Build history of the part. All positions in model axes, mm. Face numbers are marked on the shaded views. A direction names the side the tool comes from. Round coordinates to 2 decimals unless told otherwise and drop trailing zeros. Write each loop counter-clockwise with the first axis right and the second up, starting at its lowest first coordinate (ties: lowest second). Pieces come first, ordered by that corner, then holes.
Item 1: Drop flat-ended pins along their axis: pin 1 Ø1.5 at (y, z) = (11.5, 3) entering from -X; pin 2 Ø12 at (x, y) = (3, 0) entering from -Z; pin 3 Ø1.5 at (y, z) = (10, 2.5) entering from +X; pin 4 Ø1.5 at (x, y) = (11, -4) entering from +Z. Give the stop position or say it passes through.
Item 2: Wall check: probe 1 along Y at (x, z) = (-10, 2.1); probe 2 along Y at (x, z) = (-8, 0.4); probe 3 along X at (y, z) = (-10, 2.45). Give the ranges that are in metal, low to high.
Item 3: Band-saw the part on C-C, the plane x = 22.5. Write the cut outline in (y, z).
Item 4: Band-saw the part on A-A, the plane y = -9.5. Write the cut outline in (x, z).
Item 5: 3-axis set-ups, long thin cutter, end or side, ignore diameter. For the marked faces 4 and 5: which of +Z, -Z, +X, -X, +Y, -Y reach the whole face in a straight line?
Item 6: Band-saw the part on B-B, the plane x = 6. Write the cut outline in (y, z), then the cut area to 3 significant figures.
Item 7: Mould opens along X. For the marked faces 1, 2 and 3 say: +X half, -X half, draft (parallel to the pull), parting line (faces both ways), or undercut.
Item 8: Band-saw the part on D-D, the plane z = 2.5. Count the separate pieces of the cut face and the enclosed holes in it, then the cut area to 3 significant figures.
```python
from build123d import *

# Parameters (mm, degrees)
SKETCH1_W                 = 42
SKETCH1_H                 = 43
BOSS_EXTRUDE1_DEPTH       = 5
SKETCH2_W                 = 31.6
SKETCH2_H                 = 12.6
CUT_EXTRUDE1_DEPTH        = 3
SKETCH3_W                 = 25.6
SKETCH3_H                 = 7.6
CUT_EXTRUDE2_DEPTH        = 3
CUT_EXTRUDE3_DEPTH        = 5
SKETCH5_W                 = 5
SKETCH5_H                 = 5
BOSS_EXTRUDE2_DEPTH       = 5
SKETCH6_W                 = 5
SKETCH6_H                 = 5
BOSS_EXTRUDE3_DEPTH       = 5
FILLET1_R                 = 2
FILLET2_R                 = 1
M3X0_5_TAPPED_HOLE1_D     = 2.5
M3X0_5_TAPPED_HOLE1_DEPTH = 7.5
M3X0_5_TAPPED_HOLE1_TIP   = 0.751075774


with BuildPart() as part:
    # Sketch1 → Boss-Extrude1 (new body)
    with BuildSketch(Plane.XY):
        Rectangle(SKETCH1_W, SKETCH1_H)
    extrude(amount=BOSS_EXTRUDE1_DEPTH)

    # Sketch2 → Cut-Extrude1 (cut)
    with BuildSketch(Plane.XY.offset(5)):
        with Locations((-0.5, 10)):
            Rectangle(SKETCH2_W, SKETCH2_H)
        with Locations((-0.5, -8.6)):
            Rectangle(SKETCH2_W, SKETCH2_H)
    extrude(amount=-CUT_EXTRUDE1_DEPTH, mode=Mode.SUBTRACT)

    # Sketch3 → Cut-Extrude2 (cut)
    with BuildSketch(Plane.XY.offset(2)):
        with Locations((-0.5, 10)):
            Rectangle(SKETCH3_W, SKETCH3_H)
        with Locations((-0.5, -8.6)):
            Rectangle(SKETCH3_W, SKETCH3_H)
    extrude(amount=-CUT_EXTRUDE2_DEPTH, mode=Mode.SUBTRACT)

    # Sketch4 → Cut-Extrude3 (cut)
    with BuildSketch(Plane(origin=(0, 0, 0), x_dir=(-1, 0, 0), z_dir=(0, 0, -1))):
        Polygon((-15.288574128, 21.5), (-21, 21.5), (-21, 16.307906388), (-21, -16.83473783), (-21, -21.5), (-15.288574128, -21.5), (16.313805872, -21.5), (21, -21.5), (21, -17.4), (-20, -17.4), (-20, 17.8), (21, 17.8), (21, 21.5), (16.313805872, 21.5), align=None)
    extrude(amount=-CUT_EXTRUDE3_DEPTH, mode=Mode.SUBTRACT)

    # Sketch5 → Boss-Extrude2 (add)
    with BuildSketch(Plane(origin=(20, 0, 0), x_dir=(0, 0, -1), z_dir=(1, 0, 0))):
        with Locations((-2.5, -10.3)):
            Rectangle(SKETCH5_W, SKETCH5_H)
    extrude(amount=BOSS_EXTRUDE2_DEPTH)

    # Sketch6 → Boss-Extrude3 (add)
    with BuildSketch(Plane.ZY.offset(21)):
        with Locations((2.5, -10.3)):
            Rectangle(SKETCH6_W, SKETCH6_H)
    extrude(amount=BOSS_EXTRUDE3_DEPTH)

    # Fillet1
    fillet1_edges = [part.edges().sort_by_distance(p)[0] for p in [
        (-16.3, 3.7, 3.5),
        (-16.3, 16.3, 3.5),
        (15.3, 16.3, 3.5),
        (15.3, 3.7, 3.5),
        (-16.3, -14.9, 3.5),
        (-16.3, -2.3, 3.5),
        (15.3, -2.3, 3.5),
        (15.3, -14.9, 3.5),
        (-13.3, 6.2, 1),
        (-13.3, 13.8, 1),
        (12.3, 13.8, 1),
        (12.3, 6.2, 1),
        (-13.3, -12.4, 1),
        (-13.3, -4.8, 1),
        (12.3, -4.8, 1),
        (12.3, -12.4, 1),
        (20, 17.8, 2.5),
        (20, -17.4, 2.5),
        (-21, -17.4, 2.5),
        (-21, 17.8, 2.5),
    ]]
    fillet(fillet1_edges, radius=FILLET1_R)

    # Fillet2
    fillet2_edges = [part.edges().sort_by_distance(p)[0] for p in [
        (25, -10.3, 0),
        (25, -10.3, 5),
        (-26, -10.3, 0),
        (-26, -10.3, 5),
    ]]
    fillet(fillet2_edges, radius=FILLET2_R)

    # M3x0.5 Tapped Hole1
    with Locations(Plane(origin=(-23.5, -12.8, 2.5), x_dir=(-1, 0, 0), z_dir=(0, -1, 0))):
        with Locations((0, 0), (-46, 0)):
            Hole(M3X0_5_TAPPED_HOLE1_D / 2, depth=M3X0_5_TAPPED_HOLE1_DEPTH)
            with Locations((0, 0, -(M3X0_5_TAPPED_HOLE1_DEPTH + M3X0_5_TAPPED_HOLE1_TIP / 2))):  # 118° drill point
                Cone(0, M3X0_5_TAPPED_HOLE1_D / 2, M3X0_5_TAPPED_HOLE1_TIP, mode=Mode.SUBTRACT)


solid = part.part
```
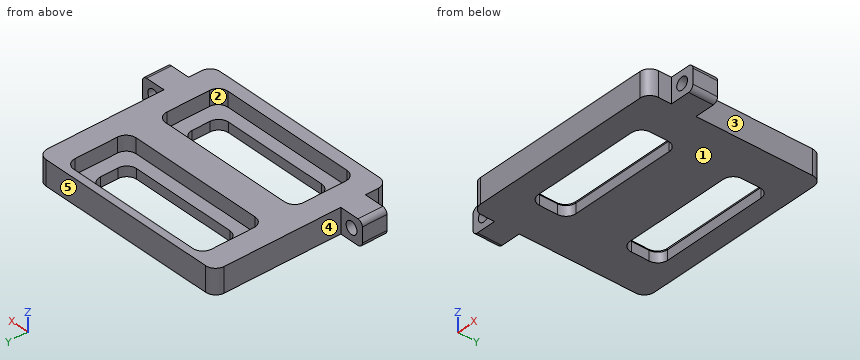
Results:
1. pin 1: stops at x = -21
1. pin 2: stops at z = 0
1. pin 3: stops at x = 20
1. pin 4: stops at z = 2
2. probe 1: y = -17.4 to -14.9, -2.3 to 3.7, 16.3 to 17.8
2. probe 2: y = -17.4 to -12.4, -4.8 to 6.2, 13.8 to 17.8
2. probe 3: x = -26 to -24.75, -22.25 to -16.3, 15.3 to 21.25, 23.75 to 25
3. outline: (-12.8, 0) - (-7.8, 0) - (-7.8, 1.25) - (-12.8, 1.25) - close; (-12.8, 3.75) - (-7.8, 3.75) - (-7.8, 5) - (-12.8, 5) - close
4. outline: (-26, 1) arc R1 ccw to (-25, 0) - (-13.3, 0) - (-13.3, 2) - (-16.3, 2) - (-16.3, 5) - (-25, 5) arc R1 ccw to (-26, 4) - close; (12.3, 0) - (24, 0) arc R1 ccw to (25, 1) - (25, 4) arc R1 ccw to (24, 5) - (15.3, 5) - (15.3, 2) - (12.3, 2) - close; hole circle Ø2.5 at (-23.5, 2.5); hole circle Ø2.5 at (22.5, 2.5)
5. face 4: +Z, -Z, -X, +Y
5. face 5: +Z, -Z, +X, -X, +Y
6. outline: (-17.4, 0) - (-12.4, 0) - (-12.4, 2) - (-14.9, 2) - (-14.9, 5) - (-17.4, 5) - close; (-4.8, 0) - (6.2, 0) - (6.2, 2) - (3.7, 2) - (3.7, 5) - (-2.3, 5) - (-2.3, 2) - (-4.8, 2) - close; (13.8, 0) - (17.8, 0) - (17.8, 5) - (16.3, 5) - (16.3, 2) - (13.8, 2) - close
6. area: 70.0 mm2
7. face 1: draft
7. face 2: undercut
7. face 3: +X half
8. separate pieces: 3
8. enclosed holes: 2
8. area: 675 mm2
